Part model, mm, in its own coordinate system. Give positions to 0.01 mm unless a question says otherwise; leave off trailing zeros. Write each loop counter-clockwise with the first axis right and the second up, starting at its lowest first coordinate (ties: lowest second). Pieces come first, ordered by that corner, then holes. Notation, with made-up numbers: M -6.5,70.25 L 40.5,70.25 A26 ccw 40.5,97.25 Z; hole C 3.5,41.5 d2. An arc over 180 degrees is marked long. Use CSV: the item, a comma, the result in double quotes. Start each with the question number.
Item 1: Cut at A-A (x = 63.5). List the corners of the cut face in (y, z).
Item 2: Cut at B-B (y = 38.1). List the corners of the cut face in (x, z), then the cut area to 3 significant figures.
Item 3: Cut at D-D (z = -0.1). List the corners of the cut face in (x, y), then the cut area to 3 significant figures.
Item 4: Pin check, flat tips, straight feed: pin 1 (1 mm diameter, centred on x = 58.5, z = -1, fed in from +Y); pin 2 (1.5 mm diameter, centred on x = 60, z = -1, fed in from +Y). Stop position of each tip, or through.
Item 5: Cut at C-C (x = 38.1). List the corners of the cut face in (y, z), then the cut area to 3 significant figures.
Item 6: Drill centre lines: line 1 (X direction, y = 12.5, z = -0.7); line 2 (Y direction, x = 63.5, z = 0.9). Where is each one in solid material? Low to high. Write a range as [from, to].
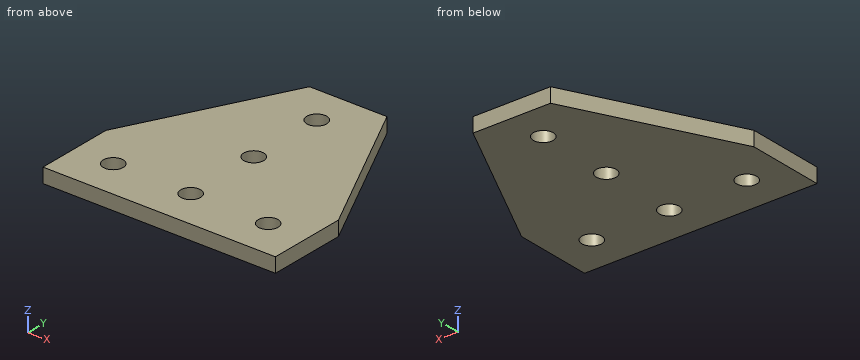
from build123d import *

# Parameters (mm, degrees)
SKETCH1_R           = 3.2639
BOSS_EXTRUDE1_DEPTH = 2.38125


with BuildPart() as part:
    # Sketch1 → Boss-Extrude1 (new body, symmetric)
    with BuildSketch(Plane.XY):
        Polygon((0, 0), (0, 25.4), (25.4, 76.2), (50.8, 76.2), (76.2, 25.4), (76.2, 0), align=None)
        with Locations((12.7, 12.7)):
            Circle(SKETCH1_R, mode=Mode.SUBTRACT)
        with Locations((38.1, 12.7)):
            Circle(SKETCH1_R, mode=Mode.SUBTRACT)
        with Locations((63.5, 12.7)):
            Circle(SKETCH1_R, mode=Mode.SUBTRACT)
        with Locations((38.1, 38.1)):
            Circle(SKETCH1_R, mode=Mode.SUBTRACT)
        with Locations((38.1, 63.5)):
            Circle(SKETCH1_R, mode=Mode.SUBTRACT)
    extrude(amount=BOSS_EXTRUDE1_DEPTH, both=True)


solid = part.part
Worked answers:
1,outline,"M 0,-2.38 L 9.44,-2.38 L 9.44,2.38 L 0,2.38 Z; M 15.96,-2.38 L 50.8,-2.38 L 50.8,2.38 L 15.96,2.38 Z"
2,outline,"M 6.35,-2.38 L 34.84,-2.38 L 34.84,2.38 L 6.35,2.38 Z; M 41.36,-2.38 L 69.85,-2.38 L 69.85,2.38 L 41.36,2.38 Z"
2,area,"271 mm^2"
3,outline,"M 0,0 L 76.2,0 L 76.2,25.4 L 50.8,76.2 L 25.4,76.2 L 0,25.4 Z; hole C 12.7,12.7 d6.53; hole C 38.1,12.7 d6.53; hole C 38.1,38.1 d6.53; hole C 38.1,63.5 d6.53; hole C 63.5,12.7 d6.53"
3,area,"4,350 mm^2"
4,pin 1,"stops at y = 61.8"
4,pin 2,"stops at y = 59.3"
5,outline,"M 0,-2.38 L 9.44,-2.38 L 9.44,2.38 L 0,2.38 Z; M 15.96,-2.38 L 34.84,-2.38 L 34.84,2.38 L 15.96,2.38 Z; M 41.36,-2.38 L 60.24,-2.38 L 60.24,2.38 L 41.36,2.38 Z; M 66.76,-2.38 L 76.2,-2.38 L 76.2,2.38 L 66.76,2.38 Z"
5,area,"270 mm^2"
6,line 1,"x = [0, 9.44], [15.96, 34.84], [41.36, 60.24], [66.76, 76.2]"
6,line 2,"y = [0, 9.44], [15.96, 50.8]"
